Geometry check sheet. Reference: drawing and pictorial views, mm from the part's lowest x, y, z. A direction names the side the tool comes from. Round coordinates to 2 decimals unless told otherwise and drop trailing zeros. Write each loop counter-clockwise with the first axis right and the second up, starting at its lowest first coordinate (ties: lowest second). Pieces come first, ordered by that corner, then holes. Notation, with made-up numbers: (-4.75, 41.5) -> (4.25, 41.5) arc R9 cw to (4.25, 47.5) -> close; hole circle Ø5 at (79.25, 38.5). An arc over 180 degrees is marked (long way). Answer as a JSON object with one key per item and string values. Group by question number.
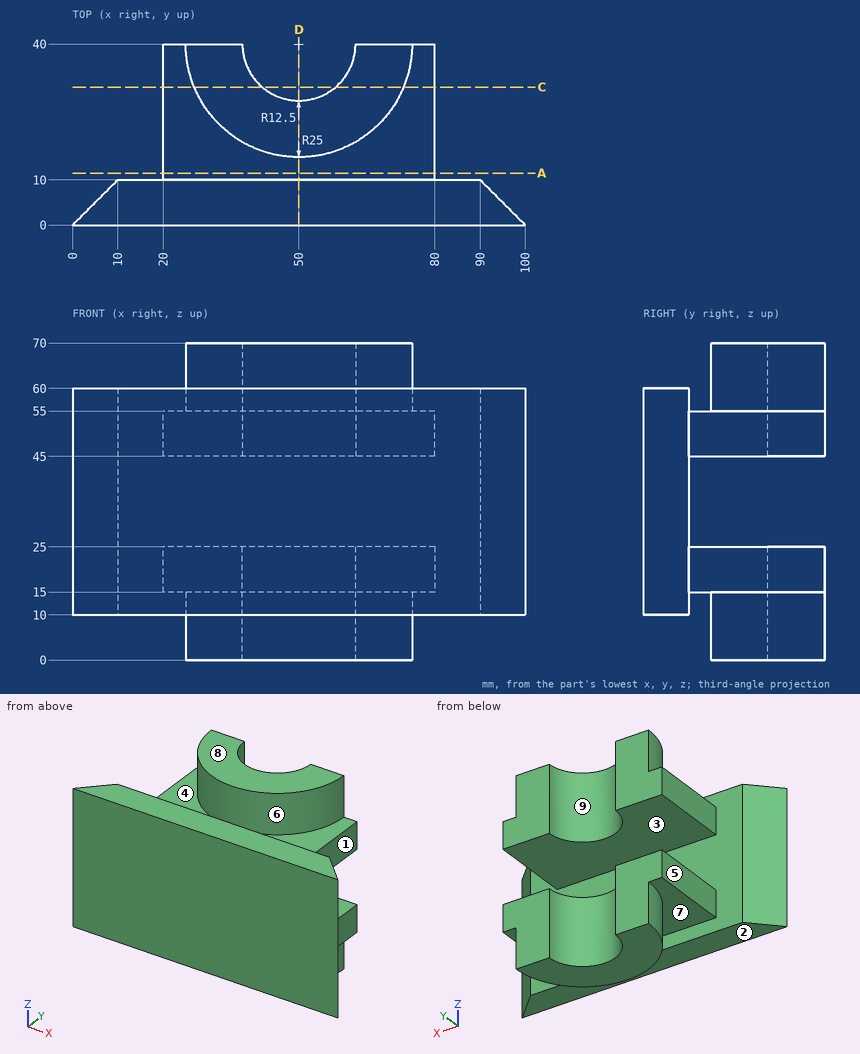
(1) Release check for a two-part mould opening along Y. For the marked faces 6, 7, 8 and 9 record: pulls with the +Y half, pulls with the -Y half, needs draft (parallel to the pull), parting line crosses it, or undercut.
(2) Access from +Z, -Z, +X, -X, +Y, -Y to the whole of each face (thin tool, end or side, straight path). Record for the marked faces 1, 2, 3, 4 and 5.
(3) Section check D-D on x = 50. Record the cut outline in (y, z), then the cut area to 4 significant figures.
(4) Go/stop test with flat-tipped pins: pin 1 Ø11 at (y, z) = (23, 47.5) entering from -X; pin 2 Ø8 at (x, y) = (20.5, 19.5) entering from -Z; pin 3 Ø2 at (x, y) = (74, 23) entering from +Z. Record where each tip stops, or that it passes through.
(5) Section check A-A on y = 11.5. Record the cut outline in (x, z), then the cut area to 3 significant figures.
(6) Scan lines: line 1 along Z through (x, y) = (27, 12.5); line 2 along X through (y, z) = (32.5, 20.5); line 3 along Z through (x, y) = (45.5, 22). Record each from-to range of solid material in increasing order.
(7) Section check C-C on y = 30.5. Record the cut outline in (x, z).
Data:
{
 "1": {"face 6": "undercut", "face 7": "undercut", "face 8": "needs draft", "face 9": "pulls with the +Y half"},
 "2": {"face 1": "+Z, -Z, +X, +Y", "face 2": "-Z, +X, -X, -Y", "face 3": "+X, -X, +Y", "face 4": "+Z", "face 5": "+Z, -Z, -X, +Y"},
 "3": {"outline": "(0, 10) -> (10, 10) -> (10, 15) -> (15, 15) -> (15, 0) -> (27.5, 0) -> (27.5, 25) -> (10, 25) -> (10, 45) -> (27.5, 45) -> (27.5, 70) -> (15, 70) -> (15, 55) -> (10, 55) -> (10, 60) -> (0, 60) -> close", "area": "1,225 mm²"},
 "4": {"pin 1": "stops at x = 20", "pin 2": "stops at z = 15", "pin 3": "stops at z = 55"},
 "5": {"outline": "(20, 15) -> (80, 15) -> (80, 25) -> (20, 25) -> close; (20, 45) -> (80, 45) -> (80, 55) -> (20, 55) -> close", "area": "1,200 mm²"},
 "6": {"line 1": "z = 15 to 25, 45 to 55", "line 2": "x = 20 to 40, 60 to 80", "line 3": "z = 0 to 25, 45 to 70"},
 "7": {"outline": "(20, 15) -> (26.88, 15) -> (26.88, 0) -> (41.88, 0) -> (41.88, 25) -> (20, 25) -> close; (20, 45) -> (41.88, 45) -> (41.88, 70) -> (26.88, 70) -> (26.88, 55) -> (20, 55) -> close; (58.12, 0) -> (73.12, 0) -> (73.12, 15) -> (80, 15) -> (80, 25) -> (58.12, 25) -> close; (58.12, 45) -> (80, 45) -> (80, 55) -> (73.12, 55) -> (73.12, 70) -> (58.12, 70) -> close"}
}
